Build history of the part. All positions in model axes, mm. Face numbers are marked on the shaded views. A direction names the side the tool comes from. Round coordinates to 2 decimals unless told otherwise and drop trailing zeros. Write each loop counter-clockwise with the first axis right and the second up, starting at its lowest first coordinate (ties: lowest second). Pieces come first, ordered by that corner, then holes. Notation, with made-up numbers: (73, -18) -> (123, -18) arc R18 cw to (123, -11) -> close; hole circle Ø9 at (-17.75, 70). An arc over 180 degrees is marked (long way). Answer in a Markdown table with one row per item.
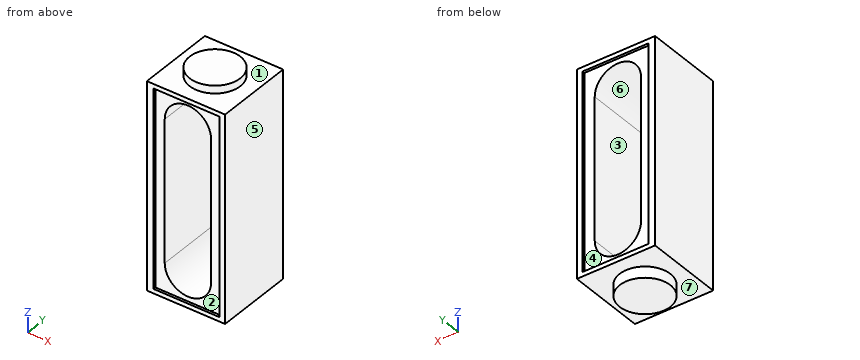
Autodesk Fusion 360 part; units mm, degrees
sketch "Sketch1" plane through (0, 0, 0) normal (0, 0, 1) x (1, 0, 0) in component "flow cell"
  circle A0 centre (0, 0) radius 9.875
  dimension "d1" = 19.75
extrude "Extrude1" add sketch "Sketch1" along normal blind 4.3 in component "flow cell"
sketch "Sketch2" plane through (0, 0, 4.3) normal (0, 0, 1) x (-1, 0, 0) in component "flow cell"
  circle A0 centre (0, 0) radius 9.875
  line L0 (12.7, 12.7) -> (-12.7, 12.7)
  line L1 (-12.7, 12.7) -> (-12.7, -12.7)
  line L2 (-12.7, -12.7) -> (12.7, -12.7)
  line L3 (12.7, -12.7) -> (12.7, 12.7)
  line L4 (12.7, 12.7) -> (-12.7, -12.7) construction
  line L5 (-12.7, 12.7) -> (12.7, -12.7) construction
  line L6 (13.7, 13.7) -> (-13.7, 13.7)
  line L7 (-13.7, 13.7) -> (-13.7, -13.7)
  line L8 (-13.7, -13.7) -> (13.7, -13.7)
  line L9 (13.7, -13.7) -> (13.7, 13.7)
  line L10 (15.2, 15.2) -> (-15.2, 15.2)
  line L11 (-15.2, 15.2) -> (-15.2, -15.2)
  line L12 (-15.2, -15.2) -> (15.2, -15.2)
  line L13 (15.2, -15.2) -> (15.2, 15.2)
  dimension "d4" = 25.4
  dimension "d5" = 25.4
  dimension "d6" = 1
  dimension "d7" = 2.5
extrude "Extrude2" add sketch "Sketch2" along normal blind 80 contours A0 | L0 L1 L2 L3 | L6 L7 L8 L9 | L10 L11 L12 L13 in component "flow cell"
sketch "Sketch3" plane through (0, 0, 84.3) normal (0, 0, 1) x (-1, 0, 0) in component "flow cell"
  line L0 (15.2, -15.2) -> (15.2, 15.2)
  line L1 (15.2, 15.2) -> (-15.2, 15.2)
  line L2 (-15.2, 15.2) -> (-15.2, -15.2)
  line L3 (-15.2, -15.2) -> (15.2, -15.2)
  circle A0 centre (0, 0) radius 9.875
  dimension "d10" = 19.75
extrude "Extrude3" add sketch "Sketch3" along normal blind 3 contours A0 in component "flow cell"
sketch "Sketch4" plane through (0, -15.2, 0) normal (0, -1, 0) x (1, 0, 0) in component "flow cell"
  line L0 (-15.2, 4.3) -> (15.2, 4.3)
  line L1 (15.2, 4.3) -> (15.2, 84.3)
  line L2 (15.2, 84.3) -> (-15.2, 84.3)
  line L3 (-15.2, 84.3) -> (-15.2, 4.3)
  line L4 (13.0604, 6) -> (-12.5396, 6)
  line L5 (-12.5396, 6) -> (-12.5396, 82.6)
  line L6 (-12.5396, 82.6) -> (13.0604, 82.6)
  line L7 (13.0604, 82.6) -> (13.0604, 6)
  line L8 (13.0604, 6) -> (-12.5396, 82.6) construction
  line L9 (-12.5396, 6) -> (13.0604, 82.6) construction
  line L10 (0.2604, 44.3) -> (-15.2, 44.3) construction
  point P0 (0.2604, 44.3)
  dimension "d13" = 25.6
  dimension "d14" = 76.6
extrude "Extrude4" cut sketch "Sketch4" against normal blind 1 contours L4 L5 L6 L7 in component "flow cell"
ref_plane "WorkPlane1" through (0, 0, 44.3) normal (0, -1, 0) x (1, 0, 0) in component "flow cell"
mirror "Mirror1" about plane through (0, 0, 44.3) normal (0, -1, 0) of "Extrude4" in component "flow cell"
sketch "Sketch5" plane through (0, -14.2, 0) normal (0, -1, 0) x (1, 0, 0) in component "flow cell"
  line L0 (13.0604, 82.6) -> (-12.5396, 82.6)
  line L1 (-12.5396, 82.6) -> (-12.5396, 6)
  line L2 (-12.5396, 6) -> (13.0604, 6)
  line L3 (13.0604, 6) -> (13.0604, 82.6)
  line L4 (-9, 71.8) -> (-9, 16.8)
  arc A0 (-9, 16.8) -> (9, 16.8) centre (0, 16.8) ccw
  line L5 (9, 16.8) -> (9, 71.8)
  arc A1 (9, 71.8) -> (-9, 71.8) centre (0, 71.8) ccw
  line L6 (0, 71.8) -> (0, 16.8) construction
  line L7 (-12.5396, 44.3) -> (0, 44.3)
  line L8 (0, 1.75) -> (0, 22.5)
  dimension "d19" = 55
  dimension "d20" = 18
extrude "Extrude5" cut sketch "Sketch5" against normal through all contours L4 A0 L5 A1 in component "flow cell"
component "flow cell" placed x (1, 0, 0) y (0, 1, 0) z (0, 0, 1) at (0, 0, 0)
Q1. Wall check: line 1 (X direction, y = 11, z = 31); line 2 (Y direction, x = 12, z = 36); line 3 (Z direction, x = -9.5, y = 12.5). Give the ranges that are in metal, low to high. Write a range as [from, to].
A:
| item | result |
|---|---|
| line 1 | [-15.2, -9], [9, 15.2] |
| line 2 | [-14.2, 14.2] |
| line 3 | [4.3, 84.3] |
Q2. Saw through at C-C on z = 50. Write the cut outline in (x, y).
A:
| item | result |
|---|---|
| outline | (-15.2, -15.2) -> (-12.54, -15.2) -> (-12.54, -14.2) -> (-9, -14.2) -> (-9, 14.2) -> (-12.54, 14.2) -> (-12.54, 15.2) -> (-15.2, 15.2) -> close; (9, -14.2) -> (13.06, -14.2) -> (13.06, -15.2) -> (15.2, -15.2) -> (15.2, 15.2) -> (13.06, 15.2) -> (13.06, 14.2) -> (9, 14.2) -> close |
Q3. Saw through at D-D on x = 11. Write the cut outline in (y, z), plus the area to 3 significant figures.
A:
| item | result |
|---|---|
| outline | (-15.2, 4.3) -> (15.2, 4.3) -> (15.2, 6) -> (14.2, 6) -> (14.2, 82.6) -> (15.2, 82.6) -> (15.2, 84.3) -> (-15.2, 84.3) -> (-15.2, 82.6) -> (-14.2, 82.6) -> (-14.2, 6) -> (-15.2, 6) -> close |
| area | 2,280 mm² |
Q4. Which spindle directions (+Z, -Z, +X, -X, +Y, -Y) get a long thin tool onto all of the face, cutting with end or side? Do the marked faces 1, 2, 3 and 4. Say none if no direction does.
A:
| item | result |
|---|---|
| face 1 | +Z |
| face 2 | -Y |
| face 3 | +Y, -Y |
| face 4 | +Y |
Q5. Saw through at B-B on y = 0. Write the cut outline in (x, z) (3 decimals), plus the area to 3 significant figures.
A:
| item | result |
|---|---|
| outline | (-15.2, 4.3) -> (-9.875, 4.3) -> (-9.875, 0) -> (9.875, 0) -> (9.875, 4.3) -> (15.2, 4.3) -> (15.2, 84.3) -> (9.875, 84.3) -> (9.875, 87.3) -> (-9.875, 87.3) -> (-9.875, 84.3) -> (-15.2, 84.3) -> close; hole (-9, 16.8) arc R9 ccw to (9, 16.8) -> (9, 71.8) arc R9 ccw to (-9, 71.8) -> close |
| area | 1,330 mm² |
Q6. Saw through at A-A on x = 0. Write the cut outline in (y, z) (3 decimals).
A:
| item | result |
|---|---|
| outline | (-15.2, 4.3) -> (-9.875, 4.3) -> (-9.875, 0) -> (9.875, 0) -> (9.875, 4.3) -> (15.2, 4.3) -> (15.2, 6) -> (14.2, 6) -> (14.2, 7.8) -> (-14.2, 7.8) -> (-14.2, 6) -> (-15.2, 6) -> close; (-15.2, 82.6) -> (-14.2, 82.6) -> (-14.2, 80.8) -> (14.2, 80.8) -> (14.2, 82.6) -> (15.2, 82.6) -> (15.2, 84.3) -> (9.875, 84.3) -> (9.875, 87.3) -> (-9.875, 87.3) -> (-9.875, 84.3) -> (-15.2, 84.3) -> close |
Q7. Drop flat-ended pins along their axis: P1, Ø3, axis at x = 11.5, y = -11, coming from the +Z side; P2, Ø1.1, axis at x = 3, y = -14.5, coming from the -Z side. Give the stop position or say it passes through.
A:
| item | result |
|---|---|
| P1 | z = 84.3 |
| P2 | z = 4.3 |
Q8. Two-plate mould, pull along X, no slides. Class the marked faces 5, 6 and 7: released by +X, released by -X, zero draft, split by the parting line, or undercut.
A:
| item | result |
|---|---|
| face 5 | released by +X |
| face 6 | undercut |
| face 7 | zero draft |
